```python
from build123d import *

# Parameters (mm, degrees)
F0_W     = 95.25
F0_H     = 76.2
F1_DEPTH = 25.4
F3_D     = 47.752
F5_D     = 7.1374


with BuildPart() as f1:
    # F0 (on Front) → F1 (new body)
    with BuildSketch(Plane.XZ):
        with Locations((3.213696, -2.745525)):
            Rectangle(F0_W, F0_H)
    extrude(amount=F1_DEPTH)

    # F3 (through all)
    with Locations(Plane.XZ.offset(25.4)):
        with Locations((0, 0)):
            Hole(F3_D / 2)

    # F5 (through all)
    with Locations(Plane.XY.offset(35.354475)):
        with Locations((-34.886304, -10.860083), (41.313696, -10.860083)):
            Hole(F5_D / 2)


solid = f1.part
```
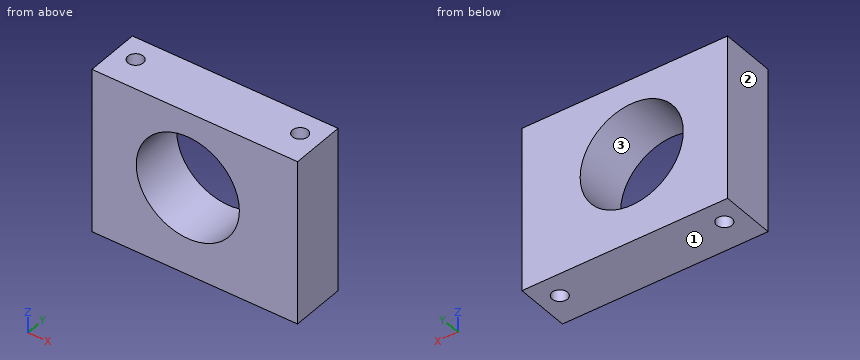
Geometry: final body of the model. Coordinates: model frame, mm. Face numbers are marked on the shaded views. Round coordinates to 2 decimals unless told otherwise and drop trailing zeros. Loops run counter-clockwise (first coordinate to the right, second up) from the corner with the lowest first, then second, coordinate; pieces in that order, holes last. Notation, with made-up numbers: (72.5, -20) -> (94.5, -20) arc R29 ccw to (94.5, 18) -> close; hole circle Ø1 at (38, 89.5). An arc over 180 degrees is marked (long way). Use one line per item in the form item = value.
Item 1: Cut plane A-A on x = 0. Output: boundary loops of the cut face in (y, z).
Evaluation:
outline = (-25.4, -40.85) -> (0, -40.85) -> (0, -23.88) -> (-25.4, -23.88) -> close; (-25.4, 23.88) -> (0, 23.88) -> (0, 35.35) -> (-25.4, 35.35) -> close
Item 2: Cut plane D-D on z = -8. Output: boundary loops of the cut face in (x, y) (3 decimals).
Evaluation:
outline = (-44.411, -25.4) -> (-22.496, -25.4) -> (-22.496, 0) -> (-44.411, 0) -> close; (22.496, -25.4) -> (50.839, -25.4) -> (50.839, 0) -> (22.496, 0) -> close; hole circle Ø7.137 at (-34.886, -10.86); hole circle Ø7.137 at (41.314, -10.86)
Item 3: Draft query along Z for the marked faces 1, 2 and 3. Return one class per face: released by +Z, released by -Z, zero draft, split by the parting line, or undercut.
Evaluation:
face_1 = released by -Z
face_2 = zero draft
face_3 = undercut
Item 4: Material intervals for probe 1 along X at (y, z) = (-10.75, 25); probe 2 along X at (y, z) = (-13.25, 2); probe 3 along X at (y, z) = (-13.75, -11.5), sorted ascending.
Evaluation:
probe_1 = -44.41 to -38.45, -31.32 to 37.75, 44.88 to 50.84
probe_2 = -44.41 to -37.54, -32.24 to -23.79, 23.79 to 38.66, 43.96 to 50.84
probe_3 = -44.41 to -36.98, -32.79 to -20.92, 20.92 to 39.22, 43.41 to 50.84
Item 5: Cut plane C-C on y = -4.5. Output: boundary loops of the cut face in (x, z), then the cut area to 3 significant figures.
Evaluation:
outline = (-44.41, -40.85) -> (50.84, -40.85) -> (50.84, 35.35) -> (-44.41, 35.35) -> close; hole circle Ø47.75 at (0, 0)
area = 5,470 mm2
Item 6: Cut plane B-B on z = 0. Output: boundary loops of the cut face in (x, y) (3 decimals), then the cut area to 3 significant figures.
Evaluation:
outline = (-44.411, -25.4) -> (-23.876, -25.4) -> (-23.876, 0) -> (-44.411, 0) -> close; (23.876, -25.4) -> (50.839, -25.4) -> (50.839, 0) -> (23.876, 0) -> close; hole circle Ø7.137 at (-34.886, -10.86); hole circle Ø7.137 at (41.314, -10.86)
area = 1,130 mm2
